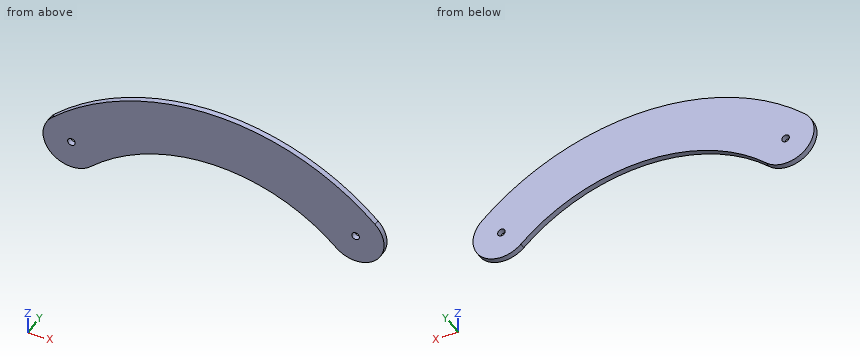
from build123d import *

# Parameters (mm, degrees)
F1_R     = 2
F2_DEPTH = 1.5


with BuildPart() as f2:
    # F1 (on Front) → F2 (new body, symmetric)
    with BuildSketch(Plane.XZ):
        with BuildLine():
            ThreePointArc((-64.7408830668, -10.9430580621), (0, 14.6585609973), (64.7408830668, -10.9430580621))
            ThreePointArc((64.7408830668, -10.9430580621), (85.9430580621, -10.2591169332), (85.2591169332, 10.9430580621))
            ThreePointArc((85.2591169332, 10.9430580621), (0, 44.6585609973), (-85.2591169332, 10.9430580621))
            ThreePointArc((-85.2591169332, 10.9430580621), (-85.9430580621, -10.2591169332), (-64.7408830668, -10.9430580621))
        make_face()
        with Locations((-75, 0)):
            Circle(F1_R, mode=Mode.SUBTRACT)
        with Locations((75, 0)):
            Circle(F1_R, mode=Mode.SUBTRACT)
    extrude(amount=F2_DEPTH, both=True)


solid = f2.part
Work out the finished part from the listing and answer in its coordinate system (mm). Give positions to 0.01 mm unless a question says otherwise; leave off trailing zeros. Loops run counter-clockwise (first coordinate to the right, second up) from the corner with the lowest first, then second, coordinate; pieces in that order, holes last. Notation, with made-up numbers: (45.25, 73) -> (94.25, 73) arc R28 ccw to (94.25, 110) -> close; hole circle Ø1 at (-37.5, 39.25). An arc over 180 degrees is marked (long way). Use a Markdown table: item, result. Add a question column.
1. Section B-B on z = 0 is taken. Determine the outline of the cut face in (x, y), and give its area (3 significant figures).
2. Flat-ended cylindrical pins translate along their axes: pin 1 Ø2.5 at (x, z) = (-75, 0) entering from -Y; pin 2 Ø1.5 at (y, z) = (-1, 35.5) entering from +X; pin 3 Ø1.5 at (y, z) = (-1, 5.5) entering from +X. Find the tip coordinate at first contact, or state that the pin passes through.
3. Section C-C on x = -75 is taken. Determine the outline of the cut face in (y, z), and give its area (3 significant figures).
4. Find the intervals of material crossed by probe 1 along Z at (x, y) = (-75, 0.5); probe 2 along X at (y, z) = (0.75, -5); probe 3 along X at (y, z) = (1.15, 19), in increasing order.
5. Section D-D on y = 0.3 is taken. Determine the outline of the cut face in (x, z), and give its area (3 significant figures).
6. Section A-A on z = 9 is taken. Determine the outline of the cut face in (x, y).
Results below:
| question | item | result |
|---|---|---|
| 1 | outline | (-90, -1.5) -> (-77, -1.5) -> (-77, 1.5) -> (-90, 1.5) -> close; (-73, -1.5) -> (-50.6, -1.5) -> (-50.6, 1.5) -> (-73, 1.5) -> close; (50.6, -1.5) -> (73, -1.5) -> (73, 1.5) -> (50.6, 1.5) -> close; (77, -1.5) -> (90, -1.5) -> (90, 1.5) -> (77, 1.5) -> close |
| 1 | area | 212 mm^2 |
| 2 | pin 1 | passes through |
| 2 | pin 2 | stops at x = 48.71 |
| 2 | pin 3 | stops at x = 89.23 |
| 3 | outline | (-1.5, -15) -> (1.5, -15) -> (1.5, -2) -> (-1.5, -2) -> close; (-1.5, 2) -> (1.5, 2) -> (1.5, 19.57) -> (-1.5, 19.57) -> close |
| 3 | area | 91.7 mm^2 |
| 4 | probe 1 | z = -15 to -2, 2 to 19.57 |
| 4 | probe 2 | x = -89.14 to -57.75, 57.75 to 89.14 |
| 4 | probe 3 | x = -75.75 to 75.75 |
| 5 | outline | (-85.26, 10.94) arc R15 ccw to (-64.74, -10.94) arc R94.66 cw to (64.74, -10.94) arc R15 ccw to (85.26, 10.94) arc R124.66 ccw to start; hole circle Ø4 at (-75, 0); hole circle Ø4 at (75, 0) |
| 5 | area | 5,640 mm^2 |
| 6 | outline | (-87, -1.5) -> (-32.24, -1.5) -> (-32.24, 1.5) -> (-87, 1.5) -> close; (32.24, -1.5) -> (87, -1.5) -> (87, 1.5) -> (32.24, 1.5) -> close |
